```python
from build123d import *

# Parameters (mm, degrees)
BOSS_EXTRUDE1_DEPTH                    = 14.2875
F_97_0_0059_DIAMETER_HOLE1_D           = 3.175
F_97_0_0059_DIAMETER_HOLE1_CSINK_D     = 4.7625
F_97_0_0059_DIAMETER_HOLE1_CSINK_ANGLE = 100
CUT_EXTRUDE1_DEPTH                     = 12.065


with BuildPart() as part:
    # Sketch1 → Boss-Extrude1 (new body)
    with BuildSketch(Plane(origin=(0, 0, 0), x_dir=(1, 0, 0), z_dir=(0, 1, 0))):
        with BuildLine():
            Line((6.35, 0), (117.475, 0))
            ThreePointArc((117.475, 0), (121.965128061, 1.859871939), (123.825, 6.35))
            Line((123.825, 6.35), (123.825, 72.39))
            ThreePointArc((123.825, 72.39), (121.965128061, 76.880128061), (117.475, 78.74))
            Line((117.475, 78.74), (6.35, 78.74))
            ThreePointArc((6.35, 78.74), (1.859871939, 76.880128061), (0, 72.39))
            Line((0, 72.39), (0, 6.35))
            ThreePointArc((0, 6.35), (1.859871939, 1.859871939), (6.35, 0))
        make_face()
    extrude(amount=BOSS_EXTRUDE1_DEPTH)

    # #97 (0.0059) Diameter Hole1 (through all)
    with Locations(Plane(origin=(0, 14.2875, 0), x_dir=(1, 0, 0), z_dir=(0, 1, 0))):
        with Locations((5.08, 5.08), (5.08, 73.66), (118.745, 73.66), (118.745, 5.08)):
            CounterSinkHole(F_97_0_0059_DIAMETER_HOLE1_D / 2, F_97_0_0059_DIAMETER_HOLE1_CSINK_D / 2, counter_sink_angle=F_97_0_0059_DIAMETER_HOLE1_CSINK_ANGLE)

    # Sketch5 → Cut-Extrude1 (cut)
    with BuildSketch(Plane(origin=(0, 0, 0), x_dir=(-1, 0, 0), z_dir=(0, -1, 0))):
        with BuildLine():
            Line((-111.125, 73.18375), (-111.125, 62.865))
            ThreePointArc((-111.125, 62.865), (-112.984871939, 58.374871939), (-117.475, 56.515))
            Line((-117.475, 56.515), (-118.26875, 56.515))
            Line((-118.26875, 56.515), (-118.26875, 12.7))
            Line((-118.26875, 12.7), (-117.475, 12.7))
            ThreePointArc((-117.475, 12.7), (-112.984871939, 10.840128061), (-111.125, 6.35))
            Line((-111.125, 6.35), (-111.125, 5.55625))
            Line((-111.125, 5.55625), (-12.7, 5.55625))
            Line((-12.7, 5.55625), (-12.7, 15.875))
            ThreePointArc((-12.7, 15.875), (-10.840128061, 20.365128061), (-6.35, 22.225))
            Line((-6.35, 22.225), (-5.55625, 22.225))
            Line((-5.55625, 22.225), (-5.55625, 56.515))
            Line((-5.55625, 56.515), (-10.16, 56.515))
            ThreePointArc((-10.16, 56.515), (-11.956051224, 57.258948776), (-12.7, 59.055))
            Line((-12.7, 59.055), (-12.7, 73.18375))
            Line((-12.7, 73.18375), (-111.125, 73.18375))
        make_face()
    extrude(amount=-CUT_EXTRUDE1_DEPTH, mode=Mode.SUBTRACT)


solid = part.part
```
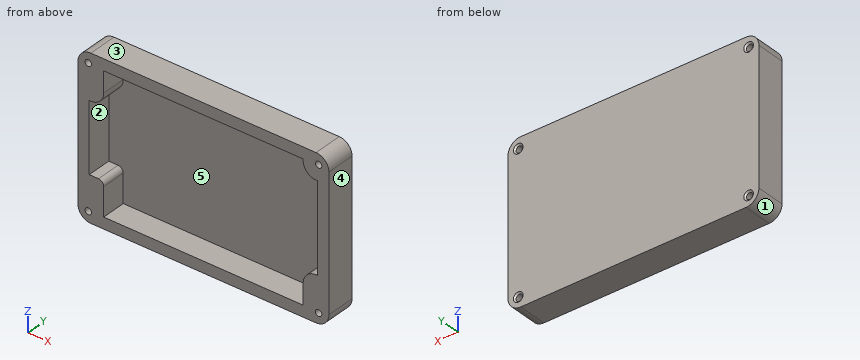
Design review of the part built by this model. Coordinates are the model's own, in mm. Face numbers are marked on the shaded views. A direction names the side the tool comes from. Coordinates: 2 decimals unless noted, no trailing zeros. Loops run counter-clockwise (first coordinate to the right, second up) from the corner with the lowest first, then second, coordinate; pieces in that order, holes last. Notation, with made-up numbers: (14, 10.5) - (57, 10.5) arc R13 ccw to (57, 18.5) - close; hole circle Ø10 at (15.5, 10.25). An arc over 180 degrees is marked (long way). Use CSV: the item, a comma, the result in double quotes. Start each with the question number.
1) For pin 1 Ø1.9 at (x, z) = (5.08, -73.66) entering from -Y; pin 2 Ø5 at (x, z) = (53, -43.5) entering from -Y (3 decimals), all flat-tipped, find the tip position at first contact; note any pin that passes through.
2) Tool access review of the marked faces 4 and 5: name each direction out of +Z, -Z, +X, -X, +Y, -Y from which nothing blocks a thin tool from reaching the whole face with its end or side.
3) Consider section A-A on y = 3.75. Give the number of separate pieces and of enclosed holes in the cut face, then the cut area to 3 significant figures.
4) Wall thickness on L1, parallel to Z at x = 83, y = 7.25; L2, parallel to X at y = 8.5, z = -64.5 (3 decimals); L3, parallel to X at y = 8.5, z = -73.66: over which ranges is each line inside the solid? List them lowest first. Write a range as from..to.
5) Consider section B-B on x = 63.5. Write out the cut boundary in (y, z) (1 decimal).
6) The part is to be moulded in two halves that separate along X. For the marked faces 1, 2 and 3, say which applies: +X half, -X half, draft (parallel to the pull), parting line (faces both ways), or undercut.
7) Consider section C-C on z = -46. Write out the cut boundary in (x, y) (1 decimal).
Geometry says:
1,pin 1,"through"
1,pin 2,"y = 12.065"
2,face 4,"+Z, -Z, +X, +Y, -Y"
2,face 5,"-Y"
3,separate pieces,"1"
3,enclosed holes,"5"
3,area,"2,440 mm^2"
4,L1,"-78.74..-73.18, -5.56..0"
4,L2,"0..12.7, 111.125..123.825"
4,L3,"0.13..3.49, 6.67..117.16, 120.33..123.7"
5,outline,"(0, -78.7) - (14.3, -78.7) - (14.3, 0) - (0, 0) - (0, -5.6) - (12.1, -5.6) - (12.1, -73.2) - (0, -73.2) - close"
6,face 1,"-X half"
6,face 2,"undercut"
6,face 3,"draft"
7,outline,"(0, 0) - (5.6, 0) - (5.6, 12.1) - (118.3, 12.1) - (118.3, 0) - (123.8, 0) - (123.8, 14.3) - (0, 14.3) - close"
